Part model, mm, in its own coordinate system. A direction names the side the tool comes from. Round coordinates to 2 decimals unless told otherwise and drop trailing zeros. Loops run counter-clockwise (first coordinate to the right, second up) from the corner with the lowest first, then second, coordinate; pieces in that order, holes last.
(1) Mould opens along Y. For faces 6 (the face through (-57.2, 40.689, 4.8)), 7 (the face through (-61.51, 33.29, 15.9)), 8 (the face through (-13, 46.786, 5)) say: +Y half, -Y half, draft (parallel to the pull), parting line (faces both ways), or undercut.
(2) Flat gauge pins, fed straight in: pin 1 (3 mm diameter, centred on x = -34, y = 51.5, fed in from -Z); pin 2 (6 mm diameter, centred on x = -55.44, z = 9.9, fed in from -Y); pin 3 (1 mm diameter, centred on y = 42, z = 13, fed in from -X); pin 4 (4 mm diameter, centred on x = -61.94, y = 48.69, fed in from +Z). Where does each tip first touch, or does it go through?
(3) Probe probe 1 along Y at (x, z) = (-29.5, 1.25); probe 2 along X at (y, z) = (34.4, 9.9); probe 3 along Y at (x, z) = (-20, 3.5). List the from-to ranges inside material, lowest first.
(4) Tool access for faces 1 (the face through (-58, 30.689, 7)), 2 (the face through (-12.441, 14, 4)), 3 (the face through (-13.641, 53, 6)), 4 (the face through (-8.641, 48, 1)), 5 (the face through (-47.941, 33, 7)): list every direction of +Z, -Z, +X, -X, +Y, -Y with a clear straight run to the whole face (end or side of a thin tool).
(5) Cut at B-B on y = 39.5. List the corners of the cut face in (x, z).
(6) Cut at D-D on x = -26. List the corners of the cut face in (y, z), then the cut area to 3 significant figures.
(7) Cut at A-A on z = 1. Count the separate pieces of the cut face and the enclosed holes in it, then the cut area to 3 significant figures.
(8) Cut at C-C on x = -0.5. List the corners of the cut face in (y, z), then the cut area to 3 significant figures.
from build123d import *

# Parameters (mm, degrees)
CROQUIS1_R                 = 1.5
SALIENTE_EXTRUIR1_DEPTH    = 2.4
CROQUIS3_W                 = 25.05
CROQUIS3_H                 = 24.65
CROQUIS3_W_2               = 22.65
CROQUIS3_H_2               = 22.25
SALIENTE_EXTRUIR2_DEPTH    = 10
CROQUIS4_W                 = 25.05
CROQUIS4_H                 = 24.65
CROQUIS4_W_2               = 17.05
CROQUIS4_H_2               = 16.65
SALIENTE_EXTRUIR3_DEPTH    = 1.2
CORTAR_EXTRUIR1_START      = -11.2
CROQUIS5_W                 = 4
CROQUIS5_H                 = 2.5
CROQUIS5_W_2               = 15.15
CROQUIS5_H_2               = 4
CROQUIS5_H_3               = 1
CORTAR_EXTRUIR1_DEPTH      = 11.2
CROQUIS6_W                 = 27.4
CROQUIS6_H                 = 20.4
CROQUIS6_W_2               = 25
CROQUIS6_H_2               = 18
SALIENTE_EXTRUIR4_DEPTH    = 1.6
CROQUIS8_W                 = 15
CROQUIS8_H                 = 15
SALIENTE_EXTRUIR5_DEPTH    = 15
CROQUIS10_R                = 5
CORTAR_EXTRUIR2_DEPTH      = 5
CORTAR_EXTRUIR3_START      = -10
CROQUIS10_2_R              = 5
CORTAR_EXTRUIR3_DEPTH      = 5
CROQUIS11_R                = 3.5
CORTAR_EXTRUIR4_DEPTH      = 5
CORTAR_EXTRUIR5_DEPTH      = 2.4
CORTAR_EXTRUIR6_DEPTH      = 10
CORTAR_EXTRUIR6_DEPTH_BACK = 2.4
CROQUIS13_W                = 10
CROQUIS13_H                = 4.5
CROQUIS14_W                = 27.4
CROQUIS14_H                = 20.4
CROQUIS14_W_2              = 20.6
CROQUIS14_H_2              = 13.6
SALIENTE_EXTRUIR6_DEPTH    = 1.2
CROQUIS15_W                = 25
CROQUIS15_H                = 18
CORTAR_EXTRUIR7_DEPTH      = 2.4
CORTAR_EXTRUIR8_START      = -5.2
CROQUIS16_W                = 3.4
CROQUIS16_H                = 8
CORTAR_EXTRUIR8_DEPTH      = 5.2
REDONDEO1_R                = 5


with BuildPart() as part:
    # Croquis1 → Saliente-Extruir1 (new body)
    with BuildSketch(Plane.XY):
        with BuildLine():
            Line((-65.940699516, 48.688511327), (-65.940699516, 17.688511327))
            ThreePointArc((-65.940699516, 17.688511327), (-64.76912664, 14.860084202), (-61.940699516, 13.688511327))
            ThreePointArc((-61.940699516, 13.688511327), (-28.440699516, 5.688511327), (5.059300484, 13.688511327))
            ThreePointArc((5.059300484, 13.688511327), (9.059300484, 17.688511327), (5.059300484, 21.688511327))
            ThreePointArc((5.059300484, 21.688511327), (-6.440699516, 33.188511327), (5.059300484, 44.688511327))
            ThreePointArc((5.059300484, 44.688511327), (9.059300484, 48.688511327), (5.059300484, 52.688511327))
            ThreePointArc((5.059300484, 52.688511327), (-28.440699516, 60.688511327), (-61.940699516, 52.688511327))
            ThreePointArc((-61.940699516, 52.688511327), (-64.76912664, 51.516938452), (-65.940699516, 48.688511327))
        make_face()
        with Locations((-61.940699516, 48.688511327)):
            Circle(CROQUIS1_R, mode=Mode.SUBTRACT)
        with Locations((5.059300484, 48.688511327)):
            Circle(CROQUIS1_R, mode=Mode.SUBTRACT)
        with Locations((5.059300484, 17.688511327)):
            Circle(CROQUIS1_R, mode=Mode.SUBTRACT)
        with Locations((-61.940699516, 17.688511327)):
            Circle(CROQUIS1_R, mode=Mode.SUBTRACT)
    extrude(amount=SALIENTE_EXTRUIR1_DEPTH)

    # Croquis3 → Saliente-Extruir2 (add)
    with BuildSketch(Plane.XY.offset(2.4)):
        with Locations((-24.965699516, 42.160543548)):
            Rectangle(CROQUIS3_W, CROQUIS3_H)
        with Locations((-24.965699516, 42.160543548)):
            Rectangle(CROQUIS3_W_2, CROQUIS3_H_2, mode=Mode.SUBTRACT)
    extrude(amount=SALIENTE_EXTRUIR2_DEPTH)

    # Croquis4 → Saliente-Extruir3 (add)
    with BuildSketch(Plane.XY.offset(12.4)):
        with Locations((-24.965699516, 42.160543548)):
            Rectangle(CROQUIS4_W, CROQUIS4_H)
        with Locations((-24.965699516, 42.160543548)):
            Rectangle(CROQUIS4_W_2, CROQUIS4_H_2, mode=Mode.SUBTRACT)
    extrude(amount=SALIENTE_EXTRUIR3_DEPTH)

    # Croquis5 → Cortar-Extruir1 (cut)
    with BuildSketch(Plane.XY.offset(13.6).offset(CORTAR_EXTRUIR1_START)):
        with Locations((-35.490699516, 48.035543548)):
            Rectangle(CROQUIS5_W, CROQUIS5_H)
        with Locations((-24.015699516, 52.485543548)):
            Rectangle(CROQUIS5_W_2, CROQUIS5_H_2)
        with Locations((-14.440699516, 36.035543548)):
            Rectangle(CROQUIS5_W, CROQUIS5_H_3)
        with Locations((-14.440699516, 48.035543548)):
            Rectangle(CROQUIS5_W, CROQUIS5_H)
    extrude(amount=CORTAR_EXTRUIR1_DEPTH, mode=Mode.SUBTRACT)

    # Croquis6 → Saliente-Extruir4 (add)
    with BuildSketch(Plane.XY.offset(2.4)):
        with Locations((-26.140699516, 17.635543548)):
            Rectangle(CROQUIS6_W, CROQUIS6_H)
        with Locations((-26.140699516, 17.635543548)):
            Rectangle(CROQUIS6_W_2, CROQUIS6_H_2, mode=Mode.SUBTRACT)
    extrude(amount=SALIENTE_EXTRUIR4_DEPTH)

    # Croquis8 → Saliente-Extruir5 (add)
    with BuildSketch(Plane.XY.offset(2.4)):
        with Locations((-55.440699516, 33.188511327)):
            Rectangle(CROQUIS8_W, CROQUIS8_H)
    extrude(amount=SALIENTE_EXTRUIR5_DEPTH)

    # Croquis10 → Cortar-Extruir2 (cut)
    with BuildSketch(Plane.XZ.offset(-25.688511327)):
        with Locations(Location((-55.440699516, 9.9, 0), (0, 0, 270))):
            Circle(CROQUIS10_R)
    extrude(amount=-CORTAR_EXTRUIR2_DEPTH, mode=Mode.SUBTRACT)

    # Croquis10<2> → Cortar-Extruir3 (cut)
    with BuildSketch(Plane.XZ.offset(-25.688511327).offset(CORTAR_EXTRUIR3_START)):
        with Locations(Location((-55.440699516, 9.9, 0), (0, 0, 270))):
            Circle(CROQUIS10_2_R)
    extrude(amount=-CORTAR_EXTRUIR3_DEPTH, mode=Mode.SUBTRACT)

    # Croquis11 → Cortar-Extruir4 (cut)
    with BuildSketch(Plane.XZ.offset(-30.688511327)):
        with Locations(Location((-55.440699516, 9.9, 0), (0, 0, 270))):
            Circle(CROQUIS11_R)
    extrude(amount=-CORTAR_EXTRUIR4_DEPTH, mode=Mode.SUBTRACT)

    # Croquis12 → Cortar-Extruir5 (cut)
    with BuildSketch(Plane.XY.offset(2.4)):
        Polygon((-36.290699516, 53.285543548), (-13.640699516, 53.285543548), (-13.640699516, 49.285543548), (-8.640699516, 49.285543548), (-8.640699516, 46.785543548), (-13.640699516, 46.785543548), (-13.640699516, 31.035543548), (-36.290699516, 31.035543548), (-36.290699516, 46.785543548), (-41.290699516, 46.785543548), (-41.290699516, 49.285543548), (-36.290699516, 49.285543548), align=None)
    extrude(amount=-CORTAR_EXTRUIR5_DEPTH, mode=Mode.SUBTRACT)

    # Croquis13 → Cortar-Extruir6 (cut, two sides: drawn at the far end of the back side and taken through both)
    with BuildSketch(Plane.XY.offset(2.4).offset(-CORTAR_EXTRUIR6_DEPTH_BACK)):
        with Locations((-18.640699516, 55.535543548)):
            Rectangle(CROQUIS13_W, CROQUIS13_H)
    extrude(amount=CORTAR_EXTRUIR6_DEPTH + CORTAR_EXTRUIR6_DEPTH_BACK, mode=Mode.SUBTRACT)

    # Croquis14 → Saliente-Extruir6 (add)
    with BuildSketch(Plane.XY.offset(4)):
        with Locations((-26.140699516, 17.635543548)):
            Rectangle(CROQUIS14_W, CROQUIS14_H)
        with Locations((-26.140699516, 17.635543548)):
            Rectangle(CROQUIS14_W_2, CROQUIS14_H_2, mode=Mode.SUBTRACT)
    extrude(amount=SALIENTE_EXTRUIR6_DEPTH)

    # Croquis15 → Cortar-Extruir7 (cut)
    with BuildSketch(Plane.XY.offset(2.4)):
        with Locations((-26.140699516, 17.635543548)):
            Rectangle(CROQUIS15_W, CROQUIS15_H)
    extrude(amount=-CORTAR_EXTRUIR7_DEPTH, mode=Mode.SUBTRACT)

    # Croquis16 → Cortar-Extruir8 (cut)
    with BuildSketch(Plane.XY.offset(5.2).offset(CORTAR_EXTRUIR8_START)):
        with Locations((-14.140699516, 23.835543548)):
            Rectangle(CROQUIS16_W, CROQUIS16_H)
    extrude(amount=CORTAR_EXTRUIR8_DEPTH, mode=Mode.SUBTRACT)

    # Redondeo1
    redondeo1_edges = [part.edges().sort_by_distance(p)[0] for p in [
        (-62.940699516, 33.188511327, 17.4),
        (-47.940699516, 33.188511327, 17.4),
    ]]
    fillet(redondeo1_edges, radius=REDONDEO1_R)


solid = part.part
Final values:
1. face 6: +Y half
1. face 7: draft
1. face 8: undercut
2. pin 1: stops at z = 12.4
2. pin 2: passes through
2. pin 3: stops at x = -37.49
2. pin 4: stops at z = 2.4
3. probe 1: y = 5.7 to 8.64, 26.64 to 31.04, 53.29 to 60.68
3. probe 2: x = -62.94 to -58.94, -51.94 to -47.94, -37.49 to -36.29, -13.64 to -12.44
3. probe 3: y = 7.44 to 8.64, 26.64 to 27.84, 29.84 to 31.04
4. face 1: -Y
4. face 2: +Z, +X, +Y, -Y
4. face 3: -Z
4. face 4: +Z, -Z
4. face 5: +Z, +Y, -Y
5. outline: (-65.94, 0) - (-36.29, 0) - (-36.29, 12.4) - (-33.49, 12.4) - (-33.49, 13.6) - (-37.49, 13.6) - (-37.49, 2.4) - (-47.94, 2.4) - (-47.94, 12.4) arc R5 ccw to (-52.94, 17.4) - (-57.94, 17.4) arc R5 ccw to (-62.94, 12.4) - (-62.94, 2.4) - (-65.94, 2.4) - close; (-16.44, 12.4) - (-13.64, 12.4) - (-13.64, 0) - (-4.55, 0) - (-4.55, 2.4) - (-12.44, 2.4) - (-12.44, 13.6) - (-16.44, 13.6) - close; hole circle Ø10 at (-55.44, 9.9)
6. outline: (5.73, 0) - (8.64, 0) - (8.64, 4) - (10.84, 4) - (10.84, 5.2) - (7.44, 5.2) - (7.44, 2.4) - (5.73, 2.4) - close; (24.44, 4) - (26.64, 4) - (26.64, 0) - (31.04, 0) - (31.04, 12.4) - (33.84, 12.4) - (33.84, 13.6) - (29.84, 13.6) - (29.84, 2.4) - (27.84, 2.4) - (27.84, 5.2) - (24.44, 5.2) - close; (53.29, 0) - (60.65, 0) - (60.65, 2.4) - (53.29, 2.4) - close
6. area: 64.0 mm2
7. separate pieces: 1
7. enclosed holes: 6
7. area: 2,260 mm2
8. outline: (11.15, 0) - (23.12, 0) - (23.12, 2.4) - (11.15, 2.4) - close; (43.26, 0) - (55.22, 0) - (55.22, 2.4) - (43.26, 2.4) - close
8. area: 57.4 mm2
